Autodesk Inventor part; units mm, degrees
ref_plane "YZ Plane" through (0, 0, 0) normal (1, 0, 0) x (0, 1, 0)
ref_plane "XZ Plane" through (0, 0, 0) normal (0, 1, 0) x (-1, 0, 0)
ref_plane "XY Plane" through (0, 0, 0) normal (0, 0, 1) x (1, 0, 0)
sketch "스케치1" plane through (0, 0, 0) normal (0, 0, 1) x (1, 0, 0)
  line L0 (-25, 2.5) -> (-25, -2.5)
  line L1 (25, -2.5) -> (25, 2.5)
  line L2 (-25, -2.5) -> (25, -2.5)
  arc A0 (9, 11.5) -> (-9, 11.5) centre (0, 11.5) ccw
  line L3 (0, 11.5) -> (0, 8.5) construction
  line L4 (-3, 11.5) -> (-3, 8.5)
  line L5 (3, 8.5) -> (3, 11.5)
  arc A1 (3, 11.5) -> (-3, 11.5) centre (0, 11.5) ccw
  arc A2 (-3, 8.5) -> (3, 8.5) centre (0, 8.5) ccw
  line L6 (0, 20.1537) -> (0, 8.5) construction
  line L7 (-6, 18.2082) -> (-6, 8.5)
  line L8 (6, 8.5) -> (6, 18.2082)
  arc A3 (-6, 8.5) -> (6, 8.5) centre (0, 8.5) ccw
  line L9 (0, -7.1) -> (0, 25.1)
  line L10 (-9, 11.5) -> (-9, 2.5)
  line L11 (9, 11.5) -> (9, 2.5)
  line L12 (25, 2.5) -> (9, 2.5)
  line L13 (-9, 2.5) -> (-25, 2.5)
  point P0 (-25, 0)
  point P1 (0, 0)
  point P2 (0, 10)
  point P3 (0, 14.3269)
  dimension "d7" = 50
  dimension "d8" = 5
  dimension "d9" = 25
  dimension "d10" = 18
  dimension "d11" = 3
  dimension "d14" = 0
  dimension "d15" = 0
extrude "돌출1" add sketch "스케치1" along normal mid plane 30 contours L13 L10 A0 L7 A3 L9 L2 L0 | L9 A3 L8 A0 L11 L12 L1 L2
extrude "돌출2" add sketch "스케치1" along normal mid plane 26 contours L9 A2 L5 A1 A0 L8 A3 | A3 L7 A0 L9 A1 L4 A2
fillet "모깎기1" radius 5 2 edges at (9, 2.5, 0) (-9, 2.5, 0)
sketch "스케치3" plane through (0, 0, 0) normal (0, 0, 1) x (1, 0, 0)
  line L0 (-23.0758, 32.485) -> (23.2904, 32.485)
  line L1 (23.2904, 32.485) -> (23.2904, 2.5)
  line L2 (23.2904, 2.5) -> (-23.0758, 2.5)
  line L3 (-23.0758, 2.5) -> (-23.0758, 32.485)
  line L4 (-25, 2.5) -> (-14, 2.5)
  point P0 (0, 0)
  dimension "d21" = 0
extrude "돌출3" cut sketch "스케치3" along normal mid plane 20
sketch "스케치4" plane through (-25, 2.5, 15) normal (0, 1, 0) x (1, 0, 0)
  line L0 (8.5, 18.5) -> (41.5, 18.5)
  line L1 (41.5, 18.5) -> (41.5, 11.5)
  line L2 (41.5, 11.5) -> (8.5, 11.5)
  line L3 (8.5, 11.5) -> (8.5, 18.5)
  line L4 (8.5, 18.5) -> (41.5, 11.5) construction
  line L5 (41.5, 18.5) -> (8.5, 11.5) construction
  point P0 (25, 15)
  dimension "d24" = 33
  dimension "d25" = 7
extrude "돌출4" cut sketch "스케치4" against normal blind 20
fillet "모깎기2" radius 5 2 edges at (-25, 0, -15) (25, 0, 15)
fillet "모깎기3" radius 10 2 edges at (-25, 0, 15) (25, 0, -15)
properties part number "15-1"
Work out the finished part from the listing and answer in its coordinate system (mm). A direction names the side the tool comes from. Give positions to 0.01 mm unless a question says otherwise; leave off trailing zeros. Loops run counter-clockwise (first coordinate to the right, second up) from the corner with the lowest first, then second, coordinate; pieces in that order, holes last. Notation, with made-up numbers: (-22, -33.75) - (14, -33.75) arc R13 cw to (14, -29.75) - close; hole circle Ø4 at (65, 81.5). An arc over 180 degrees is marked (long way). Answer in a Markdown table with one row per item.
(1) Section B-B (y = -1) is taken. Give the vertices of the cut face in (x, z), and give its area (3 significant figures).
Results list:
| item | result |
|---|---|
| outline | (-25, -10) arc R5 ccw to (-20, -15) - (15, -15) arc R10 ccw to (25, -5) - (25, 10) arc R5 ccw to (20, 15) - (-15, 15) arc R10 ccw to (-25, 5) - close; hole (-16.5, -3.5) - (16.5, -3.5) - (16.5, 3.5) - (-16.5, 3.5) - close |
| area | 1,220 mm² |
(2) A tool of negligible diameter and unlimited length cuts with its end or side. For faces 4 (the face through (0.1, 5.5, 11.5)), 5 (the face through (9, 10, 12)), 6 (the face through (6, 13, 14)), 7 (the face through (6, 13, -14)), from which of +Z, -Z, +X, -X, +Y, -Y can it reach the whole face along a straight path? Write none if from no direction.
Results list:
| item | result |
|---|---|
| face 4 | +Z, -Z |
| face 5 | +Z, -Z, +X, +Y |
| face 6 | +Z, +Y |
| face 7 | -Z, +Y |
(3) Section D-D (y = 15.5) is taken. Give the vertices of the cut face in (x, z).
Results list:
| item | result |
|---|---|
| outline | (-8.06, -15) - (-6, -15) - (-6, -13) - (6, -13) - (6, -15) - (8.06, -15) - (8.06, -10) - (-8.06, -10) - close; (-8.06, 10) - (8.06, 10) - (8.06, 15) - (6, 15) - (6, 13) - (-6, 13) - (-6, 15) - (-8.06, 15) - close |
(4) Section A-A (z = 0.25) is taken. Give the vertices of the cut face in (x, y), and give its area (3 significant figures).
Results list:
| item | result |
|---|---|
| outline | (-25, -2.5) - (-16.5, -2.5) - (-16.5, 2.5) - (-25, 2.5) - close; (16.5, -2.5) - (25, -2.5) - (25, 2.5) - (16.5, 2.5) - close |
| area | 85.0 mm² |
(5) Flat-ended cylindrical pins translate along their axes: pin 1 Ø1 at (y, z) = (12, -13.5) entering from -X; pin 2 Ø2 at (y, z) = (14, 14.5) entering from +X; pin 3 Ø2 at (y, z) = (13, -14) entering from +X. Find the tip coordinate at first contact, or state that the pin passes through.
Results list:
| item | result |
|---|---|
| pin 1 | stops at x = -9 |
| pin 2 | stops at x = 8.87 |
| pin 3 | stops at x = 8.99 |
(6) Consider L1, parallel to X at y = 2.25, z = 0; L2, parallel to Z at x = 4, y = 10.5; L3, parallel to Z at x = 6, y = 3.5. Determine where each line is inside the solid, lowest interval first. Write a range as [from, to].
Results list:
| item | result |
|---|---|
| L1 | x = [-25, -16.5], [16.5, 25] |
| L2 | z = [-13, -10], [10, 13] |
| L3 | z = [-15, -10], [10, 15] |
(7) For a pull along X with two mould halves and no side action, classify faces 1 (the face through (9, 10, -13)), 2 (the face through (-0.198, 20.498, -11.979)), 3 (the face through (-3, 10, 11)) as pulls with the +X half, pulls with the -X half, needs draft (parallel to the pull), parting line crosses it, or undercut.
Results list:
| item | result |
|---|---|
| face 1 | pulls with the +X half |
| face 2 | parting line crosses it |
| face 3 | undercut |
(8) Section C-C (x = 1) is taken. Give the vertices of the cut face in (y, z).
Results list:
| item | result |
|---|---|
| outline | (-2.5, -15) - (2.58, -15) - (2.58, -13) - (5.67, -13) - (5.67, -10) - (2.5, -10) - (2.5, -3.5) - (-2.5, -3.5) - close; (-2.5, 3.5) - (2.5, 3.5) - (2.5, 10) - (5.67, 10) - (5.67, 13) - (2.58, 13) - (2.58, 15) - (-2.5, 15) - close; (14.33, -13) - (20.44, -13) - (20.44, -10) - (14.33, -10) - close; (14.33, 10) - (20.44, 10) - (20.44, 13) - (14.33, 13) - close |
